Can you work these out from the drawing? Everything is in mm from the part's minimum corner. A direction names the side the tool comes from. Round coordinates to 2 decimals unless told otherwise and drop trailing zeros. Order: outer loops, then holes, each group sorted by start corner. A loop starts at its lowest first (then second) coordinate and runs counter-clockwise, first axis right, second up. Notation, with made-up numbers: (32, 41.25) -> (79, 41.25) arc R17 ccw to (79, 59.25) -> close; hole circle Ø2 at (-26.75, 34). An arc over 180 degrees is marked (long way). One line per item, written item: value.
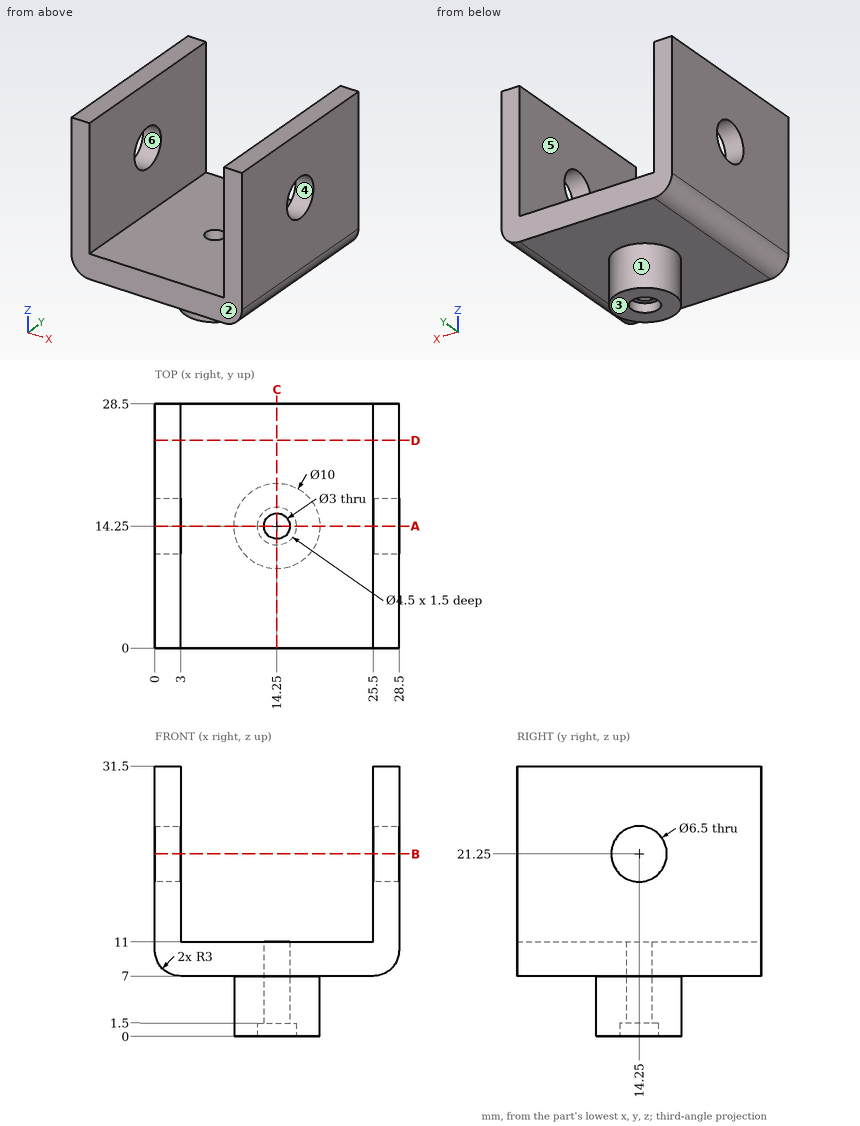
Q1. I need wall thicknesses on line 1 along X through (y, z) = (6.25, 25); line 2 along Y through (x, z) = (14.25, 7.75); line 3 along Y through (x, z) = (14.25, 0.95). Which ranges of each line are inside material? Lowest first, please.
Answers:
line 1: 0 to 3, 25.5 to 28.5
line 2: 0 to 12.75, 15.75 to 28.5
line 3: 9.25 to 12, 16.5 to 19.25
Q2. If we mould it in two halves opening along Y, with no side actions, what happens to the marked faces 1, 2, 3 and 4? For each: pulls with the +Y half, pulls with the -Y half, needs draft (parallel to the pull), parting line crosses it, or undercut.
Answers:
face 1: parting line crosses it
face 2: pulls with the -Y half
face 3: needs draft
face 4: undercut
Q3. Which directions (+Z, -Z, +X, -X, +Y, -Y) give clear straight access to the entire face, cutting with the end or side of a thin tool? Please do the marked faces 5 and 6.
Answers:
face 5: +Z, +Y, -Y
face 6: +X, -X
Q4. I want a section at A-A on y = 14.25. Give the number of separate pieces and of enclosed holes in the cut face, then the cut area to 3 significant figures.
Answers:
separate pieces: 4
enclosed holes: 0
area: 229 mm2
Q5. I want a section at D-D on y = 24.25. Write out the boundary of the cut face in (x, z).
Answers:
outline: (0, 10) arc R3 ccw to (3, 7) -> (25.5, 7) arc R3 ccw to (28.5, 10) -> (28.5, 31.5) -> (25.5, 31.5) -> (25.5, 11) -> (3, 11) -> (3, 31.5) -> (0, 31.5) -> close
Q6. I want a section at B-B on z = 21.25. Write out the boundary of the cut face in (x, y), then the cut area to 3 significant figures.
Answers:
outline: (0, 0) -> (3, 0) -> (3, 11) -> (0, 11) -> close; (0, 17.5) -> (3, 17.5) -> (3, 28.5) -> (0, 28.5) -> close; (25.5, 0) -> (28.5, 0) -> (28.5, 11) -> (25.5, 11) -> close; (25.5, 17.5) -> (28.5, 17.5) -> (28.5, 28.5) -> (25.5, 28.5) -> close
area: 132 mm2
Q7. I want a section at C-C on x = 14.25. Write out the boundary of the cut face in (y, z), then the cut area to 3 significant figures.
Answers:
outline: (0, 7) -> (9.25, 7) -> (9.25, 0) -> (12, 0) -> (12, 1.5) -> (12.75, 1.5) -> (12.75, 11) -> (0, 11) -> close; (15.75, 1.5) -> (16.5, 1.5) -> (16.5, 0) -> (19.25, 0) -> (19.25, 7) -> (28.5, 7) -> (28.5, 11) -> (15.75, 11) -> close
area: 149 mm2
Q8. For P1, Ø8, axis at x = 3.5, y = 4.5, coming from the -Z side; P2, Ø4, axis at x = 11, z = 5.5, coming from the +Y side; P3, Ø7, axis at x = 16, y = 15.5, coming from the +Z side, each with a flat end and sliding along its axis, tell me the tip position at first contact or that it passes through.
Answers:
P1: z = 7
P2: y = 28.5
P3: z = 11
